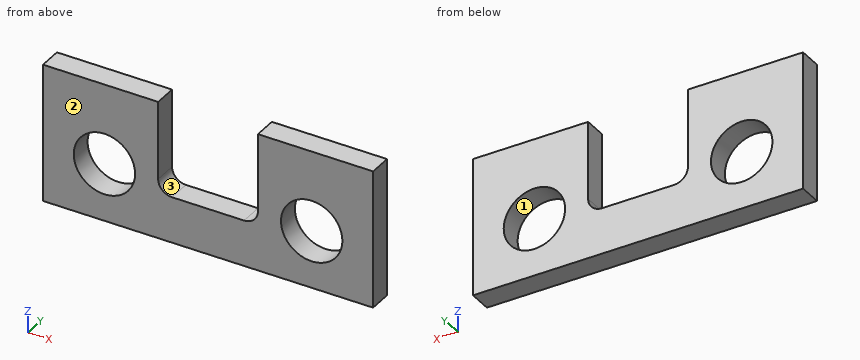
from build123d import *

# Parameters (mm, degrees)
F0_W     = 273.05
F0_H     = 114.3
F1_DEPTH = 19.05
F2_R     = 25.4
F3_DEPTH = 25.4
F5_DEPTH = 25.4


with BuildPart() as f1:
    # F0 (on Front) → F1 (new body)
    with BuildSketch(Plane.XZ):
        with Locations((136.525, 57.15)):
            Rectangle(F0_W, F0_H)
    extrude(amount=F1_DEPTH)

    # F2 (on face) → F3 (cut)
    with BuildSketch(Plane.XZ.offset(19.05)):
        with Locations((222.25, 47.625)):
            Circle(F2_R)
        with Locations((50.8, 47.625)):
            Circle(F2_R)
    extrude(amount=-F3_DEPTH, mode=Mode.SUBTRACT)

    # F4 (on face) → F5 (cut)
    with BuildSketch(Plane.XZ.offset(19.05)):
        with BuildLine():
            Line((177.8, 114.3), (95.25, 114.3))
            Line((95.25, 114.3), (95.25, 49.53))
            ThreePointArc((95.25, 49.53), (98.597769, 41.447769), (106.68, 38.1))
            Line((106.68, 38.1), (166.37, 38.1))
            ThreePointArc((166.37, 38.1), (174.452231, 41.447769), (177.8, 49.53))
            Line((177.8, 49.53), (177.8, 114.3))
        make_face()
    extrude(amount=-F5_DEPTH, mode=Mode.SUBTRACT)


solid = f1.part
Read the model definition and answer for the solid it produces. Units are mm, in the model's axes. Face numbers are marked on the shaded views. Round coordinates to 2 decimals unless told otherwise and drop trailing zeros. Loops run counter-clockwise (first coordinate to the right, second up) from the corner with the lowest first, then second, coordinate; pieces in that order, holes last.
Q1. Each of these flat-tipped pins is pushed along its axis until it touches: pin 1 (6 mm diameter, centred on x = 60.5, y = -12, fed in from -Z); pin 2 (5 mm diameter, centred on x = 165, y = -13.5, fed in from +Z); pin 3 (6 mm diameter, centred on x = 103.5, y = -5.5, fed in from +Z). Where does it stop, or does it pass through?
Q2. Section A-A on z = 83 is taken. Write down the section's boundary in (x, y).
Q3. Section B-B on x = 222.25 is taken. Write down the section's boundary in (y, z) (3 decimals), and give its area (3 significant figures).
Q4. Section C-C on y = -9.5 is taken. Write down the section's boundary in (x, z) (3 decimals), and give its area (3 significant figures).
Q5. Determine the mould class of the marked faces 1, 2 and 3 for opening direction Z: released by +Z, released by -Z, zero draft, split by the parting line, or undercut.
Q6. Section D-D on z = 65 is taken. Write down the section's boundary in (x, y), and give its area (3 significant figures).
Q7. Consider probe 1 along X at (y, z) = (-4.75, 75); probe 2 along Z at (x, y) = (222.25, -8.5) (3 decimals); probe 3 along X at (y, z) = (-2.5, 33.5). Determine where each line is inside the solid, lowest interval first.
Output:
1. pin 1: stops at z = 0
1. pin 2: stops at z = 38.16
1. pin 3: stops at z = 39.91
2. outline: (0, -19.05) - (95.25, -19.05) - (95.25, 0) - (0, 0) - close; (177.8, -19.05) - (273.05, -19.05) - (273.05, 0) - (177.8, 0) - close
3. outline: (-19.05, 0) - (0, 0) - (0, 22.225) - (-19.05, 22.225) - close; (-19.05, 73.025) - (0, 73.025) - (0, 114.3) - (-19.05, 114.3) - close
3. area: 1,210 mm2
4. outline: (0, 0) - (273.05, 0) - (273.05, 114.3) - (177.8, 114.3) - (177.8, 49.53) arc R11.43 cw to (166.37, 38.1) - (106.68, 38.1) arc R11.43 cw to (95.25, 49.53) - (95.25, 114.3) - (0, 114.3) - close; hole circle Ø50.8 at (50.8, 47.625); hole circle Ø50.8 at (222.25, 47.625)
4. area: 20,900 mm2
5. face 1: undercut
5. face 2: zero draft
5. face 3: released by +Z
6. outline: (0, -19.05) - (32.27, -19.05) - (32.27, 0) - (0, 0) - close; (69.33, -19.05) - (95.25, -19.05) - (95.25, 0) - (69.33, 0) - close; (177.8, -19.05) - (203.72, -19.05) - (203.72, 0) - (177.8, 0) - close; (240.78, -19.05) - (273.05, -19.05) - (273.05, 0) - (240.78, 0) - close
6. area: 2,220 mm2
7. probe 1: x = 0 to 95.25, 177.8 to 273.05
7. probe 2: z = 0 to 22.225, 73.025 to 114.3
7. probe 3: x = 0 to 29.69, 71.91 to 201.14, 243.36 to 273.05
